```python
from build123d import *

# Parameters (mm, degrees)
F0_R     = 17.5
F0_W     = 8.2477046886
F0_H     = 30
F0_W_2   = 8
F0_H_2   = 15
F1_DEPTH = 15
F2_R     = 2


with BuildPart() as f1:
    # F0 (on Top) → F1 (new body)
    with BuildSketch(Plane.XY):
        Polygon((25.6203956529, 17.2967884245), (-129.3796043471, 17.2967884245), (-129.3796043471, -7.7032115755), (-121.1318996584, -7.7032115755), (-111.1318996584, -7.7032115755), (-103.1318996584, -7.7032115755), (-93.1318996584, -7.7032115755), (-80.6687141383, -7.7032115755), (25.6203956529, -7.7032115755), align=None)
        with BuildLine():
            ThreePointArc((25.6203956529, -7.7032115755), (93.3121377295, 4.7967884245), (25.6203956529, 17.2967884245))
            Line((25.6203956529, 17.2967884245), (25.6203956529, -7.7032115755))
        make_face()
        with Locations((58.3121377295, 4.7967884245)):
            Circle(F0_R, mode=Mode.SUBTRACT)
        with Locations((-125.2557520027, -22.7032115755)):
            Rectangle(F0_W, F0_H)
        with Locations((-107.1318996584, -15.2032115755)):
            Rectangle(F0_W_2, F0_H_2)
        Polygon((-86.9003068984, -22.7032115755), (-80.6687141383, -7.7032115755), (-93.1318996584, -7.7032115755), align=None)
    extrude(amount=F1_DEPTH)

    # F2
    f2_edges = [f1.edges().sort_by_distance(p)[0] for p in [
        (-51.879604, 17.296788, 15),
        (-27.524159, -7.703212, 15),
        (-83.784511, -15.203212, 15),
        (-103.1319, -15.203212, 15),
        (-98.1319, -7.703212, 15),
        (-90.016103, -15.203212, 15),
        (-111.1319, -15.203212, 15),
        (-107.1319, -22.703212, 15),
        (-116.1319, -7.703212, 15),
        (-121.1319, -22.703212, 15),
        (-125.255752, -37.703212, 15),
        (-129.379604, -10.203212, 15),
        (93.312138, 4.796788, 15),
        (40.812138, 4.796788, 15),
        (25.620396, -7.703212, 7.5),
        (25.620396, 17.296788, 7.5),
        (93.312138, 4.796788, 0),
        (-129.379604, 17.296788, 7.5),
        (-51.879604, 17.296788, 0),
        (-116.1319, -7.703212, 0),
        (-111.1319, -15.203212, 0),
        (-121.1319, -22.703212, 0),
        (-103.1319, -15.203212, 0),
        (-98.1319, -7.703212, 0),
        (-90.016103, -15.203212, 0),
        (-27.524159, -7.703212, 0),
        (-107.1319, -22.703212, 0),
        (-83.784511, -15.203212, 0),
        (40.812138, 4.796788, 0),
    ]]
    fillet(f2_edges, radius=F2_R)


solid = f1.part
```
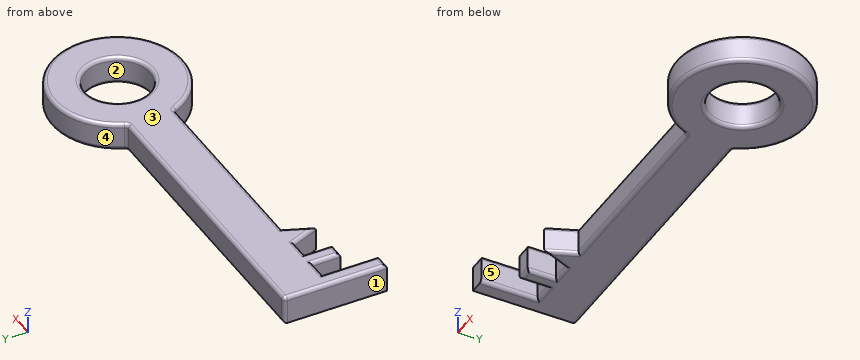
For this review, take the finished solid that the model builds, in its own axes (mm). Face numbers are marked on the shaded views. A direction names the side the tool comes from. Round coordinates to 2 decimals unless told otherwise and drop trailing zeros. Write each loop counter-clockwise with the first axis right and the second up, starting at its lowest first coordinate (ties: lowest second). Pieces come first, ordered by that corner, then holes. Notation, with made-up numbers: (74.5, -37) - (106.5, -37) arc R20 cw to (106.5, 1) - close; hole circle Ø1 at (-36.75, 89). An arc over 180 degrees is marked (long way). Answer as a JSON object with one key per item and string values.
1. We need section A-A on z = 5. Give the boundary of the cut face in (x, y), then the cut area to 3 significant figures.
Response values:
{"outline": "(-129.38, -37.7) - (-121.13, -37.7) - (-121.13, -7.7) - (-111.13, -7.7) - (-111.13, -22.7) - (-103.13, -22.7) - (-103.13, -7.7) - (-93.13, -7.7) - (-86.9, -22.7) - (-80.67, -7.7) - (24.27, -7.7) arc R2 cw to (26.11, -8.92) arc R35 ccw (long way) to (26.11, 18.51) arc R2 cw to (24.27, 17.3) - (-127.38, 17.3) arc R2 ccw to (-129.38, 15.3) - close; hole circle Ø35 at (58.31, 4.8)", "area": "7,180 mm2"}
2. Tool access review of the marked faces 4 and 5: name each direction out of +Z, -Z, +X, -X, +Y, -Y from which nothing blocks a thin tool from reaching the whole face with its end or side.
Response values:
{"face 4": "+Z, -Z", "face 5": "+Z, -Z, -Y"}
3. Draft analysis for pull direction X (two halves, no side actions). For the marked faces 1, 2 and 3, state which applies: +X half, -X half, draft (parallel to the pull), parting line (faces both ways), or undercut.
Response values:
{"face 1": "-X half", "face 2": "undercut", "face 3": "draft"}
4. To check wall thickness, follow line 1 along X through (y, z) = (-16, 6.5); line 2 along X through (y, z) = (-13, 12); line 3 along X through (y, z) = (5, 9.25). State the ranges of each line that lie inside material, in increasing order.
Response values:
{"line 1": "x = -129.38 to -121.13, -111.13 to -103.13, -89.69 to -84.12, 30.16 to 86.46", "line 2": "x = -129.38 to -121.13, -111.13 to -103.13, -90.93 to -82.87, 28.17 to 88.45", "line 3": "x = -129.38 to 40.81, 75.81 to 93.31"}
5. We need section B-B on x = 20. Give the boundary of the cut face in (y, z).
Response values:
{"outline": "(-7.7, 2) arc R2 ccw to (-5.7, 0) - (15.3, 0) arc R2 ccw to (17.3, 2) - (17.3, 13) arc R2 ccw to (15.3, 15) - (-5.7, 15) arc R2 ccw to (-7.7, 13) - close"}
6. For pin 1 Ø3.5 at (y, z) = (-15.5, 5.5) entering from +X; pin 2 Ø5 at (x, z) = (37.5, 7.5) entering from -Y; pin 3 Ø8 at (x, z) = (-99.5, 7) entering from -Y, all flat-tipped, find the tip position at first contact; note any pin that passes through.
Response values:
{"pin 1": "stops at x = 87.99", "pin 2": "stops at y = -25.03", "pin 3": "stops at y = -22.7"}
